from build123d import *

# Parameters (mm, degrees)
BOSS_EXTRUDE1_DEPTH = 2.65684
SKETCH2_R           = 12.7
CUT_EXTRUDE1_DEPTH  = 709.165228812
SKETCH3_R           = 6.35
CUT_EXTRUDE2_DEPTH  = 709.165228812


with BuildPart() as part:
    # Sketch1 → Boss-Extrude1 (new body)
    with BuildSketch(Plane(origin=(0, 0, 0), x_dir=(1, 0, 0), z_dir=(0, 1, 0))):
        Polygon((0, 450.85), (0, 0), (546.1, 0), (546.1, 25.4), align=None)
    extrude(amount=BOSS_EXTRUDE1_DEPTH)

    # Sketch2 → Cut-Extrude1 (cut, through all)
    with BuildSketch(Plane.XZ):
        with Locations(Location((254, -114.3, 0), (0, 0, 270))):
            Circle(SKETCH2_R)
    extrude(amount=-CUT_EXTRUDE1_DEPTH, mode=Mode.SUBTRACT)

    # Sketch3 → Cut-Extrude2 (cut, through all)
    with BuildSketch(Plane(origin=(0, 2.65684, 0), x_dir=(1, 0, 0), z_dir=(0, 1, 0))):
        with Locations(Location((362.072773191, 77.087559946, 0), (0, 0, 270))):
            Circle(SKETCH3_R)
        with Locations(Location((167.736694981, 39.312452986, 0), (0, 0, 270))):
            Circle(SKETCH3_R)
        with Locations(Location((232.190531828, 226.499987068, 0), (0, 0, 270))):
            Circle(SKETCH3_R)
    extrude(amount=-CUT_EXTRUDE2_DEPTH, mode=Mode.SUBTRACT)


solid = part.part
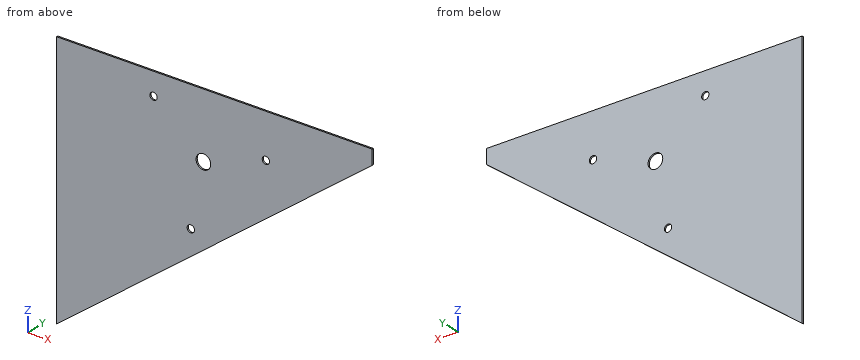
Model file for the job. Use its own axes, mm. Coordinates: 2 decimals unless noted, no trailing zeros. Write each loop counter-clockwise with the first axis right and the second up, starting at its lowest first coordinate (ties: lowest second). Pieces come first, ordered by that corner, then holes. Notation, with made-up numbers: (52, -28.75) -> (72, -28.75) arc R19 ccw to (72, -6.75) -> close; hole circle Ø3 at (-23, 50). An arc over 180 degrees is marked (long way). One line per item, written item: value. Start each with the question number.
1) Slice it at D-D on x = 400. Write the cut outline in (y, z), then the cut area to 3 significant figures.
2) Slice it at B-B on x = 254. Write the cut outline in (y, z), then the cut area to 3 significant figures.
3) Slice it at A-A on y = 1. Write the cut outline in (x, z).
4) Probe probe 1 along X at (y, z) = (1.3, -114.3); probe 2 along Z at (x, y) = (234, 0.85); probe 3 along Z at (x, y) = (486.5, 0.8). List the from-to ranges inside material, lowest first.
5) Slice it at C-C on z = -114.3. Write the cut outline in (x, y).
Answers follow:
1. outline: (0, -139.22) -> (2.66, -139.22) -> (2.66, 0) -> (0, 0) -> close
1. area: 370 mm2
2. outline: (0, -252.97) -> (2.66, -252.97) -> (2.66, -127) -> (0, -127) -> close; (0, -101.6) -> (2.66, -101.6) -> (2.66, 0) -> (0, 0) -> close
2. area: 605 mm2
3. outline: (0, -450.85) -> (546.1, -25.4) -> (546.1, 0) -> (0, 0) -> close; hole circle Ø12.7 at (167.74, -39.31); hole circle Ø12.7 at (232.19, -226.5); hole circle Ø25.4 at (254, -114.3); hole circle Ø12.7 at (362.07, -77.09)
4. probe 1: 0 to 241.3, 266.7 to 431.99
4. probe 2: -268.55 to -232.59, -220.41 to 0
4. probe 3: -71.83 to 0
5. outline: (0, 0) -> (241.3, 0) -> (241.3, 2.66) -> (0, 2.66) -> close; (266.7, 0) -> (431.99, 0) -> (431.99, 2.66) -> (266.7, 2.66) -> close
